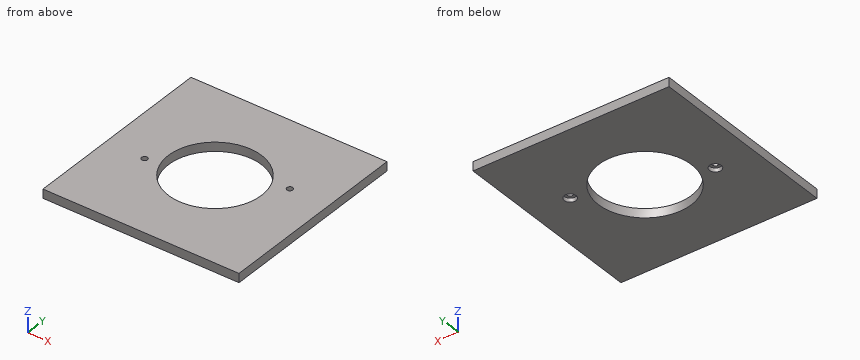
from build123d import *

# Parameters (mm, degrees)
ESQUISSE1_W             = 100
ESQUISSE1_H             = 100
ESQUISSE1_R             = 23.75
BOSS_EXTRU_1_DEPTH      = 4.6
ESQUISSE2_R             = 1.5
ENL_V_MAT_EXTRU_1_DEPTH = 10
ESQUISSE3_R             = 3
ENL_V_MAT_EXTRU_2_DEPTH = 2


with BuildPart() as part:
    # Esquisse1 → Boss.-Extru.1 (new body)
    with BuildSketch(Plane.XY):
        with Locations((5.828319543, -13.849884125)):
            Rectangle(ESQUISSE1_W, ESQUISSE1_H)
        with Locations((5.828319543, -13.849884125)):
            Circle(ESQUISSE1_R, mode=Mode.SUBTRACT)
    extrude(amount=BOSS_EXTRU_1_DEPTH)

    # Esquisse2 → Enlèv. mat.-Extru.1 (cut)
    with BuildSketch(Plane.XY.offset(4.6)):
        with Locations((-24.271680457, -21.559884125)):
            Circle(ESQUISSE2_R)
        with Locations((35.918319543, -3.129884125)):
            Circle(ESQUISSE2_R)
    extrude(amount=-ENL_V_MAT_EXTRU_1_DEPTH, mode=Mode.SUBTRACT)

    # Esquisse3 → Enlèv. mat.-Extru.2 (cut)
    with BuildSketch(Plane(origin=(0, 0, 0), x_dir=(-1, 0, 0), z_dir=(0, 0, -1))):
        with Locations((-35.918319543, -3.129884125)):
            Circle(ESQUISSE3_R)
        with Locations((24.271680457, -21.559884125)):
            Circle(ESQUISSE3_R)
    extrude(amount=-ENL_V_MAT_EXTRU_2_DEPTH, mode=Mode.SUBTRACT)


solid = part.part
Verification items for the finished model (mm, model axes). Coordinates: 2 decimals unless noted, no trailing zeros. Order: outer loops, then holes, each group sorted by start corner. A loop starts at its lowest first (then second) coordinate and runs counter-clockwise, first axis right, second up.
Item 1: Section check A-A, the plane x = -3. Enter the section's corners in (y, z).
Filled in:
outline: (-63.85, 0) - (-35.9, 0) - (-35.9, 4.6) - (-63.85, 4.6) - close; (8.2, 0) - (36.15, 0) - (36.15, 4.6) - (8.2, 4.6) - close
Item 2: Depth check by flat-ended pin: pin 1 (3.5 mm diameter, centred on x = 35.92, y = -3.13, fed in from -Z); pin 2 (1.8 mm diameter, centred on x = -24.27, y = -21.56, fed in from -Z). Enter the tip coordinate at first touch or a pass-through.
Filled in:
pin 1: stops at z = 2
pin 2: passes through
Item 3: Material ranges on L1, parallel to X at y = -14, z = 3.75; L2, parallel to Y at x = 24.5, z = 2.25; L3, parallel to X at y = -25.5, z = 0.9, recorded low to high.
Filled in:
L1: x = -44.17 to -17.92, 29.58 to 55.83
L2: y = -63.85 to -28.53, 0.83 to 36.15
L3: x = -44.17 to -14.87, 26.52 to 55.83
Item 4: Section check B-B, the plane z = 2.7. Enter the section's corners in (x, y).
Filled in:
outline: (-44.17, -63.85) - (55.83, -63.85) - (55.83, 36.15) - (-44.17, 36.15) - close; hole circle Ø3 at (-24.27, -21.56); hole circle Ø47.5 at (5.83, -13.85); hole circle Ø3 at (35.92, -3.13)
Item 5: Section check C-C, the plane y = 4.5. Enter the section's corners in (x, z), then the cut area to 3 significant figures.
Filled in:
outline: (-44.17, 0) - (-9.25, 0) - (-9.25, 4.6) - (-44.17, 4.6) - close; (20.91, 0) - (55.83, 0) - (55.83, 4.6) - (20.91, 4.6) - close
area: 321 mm2
